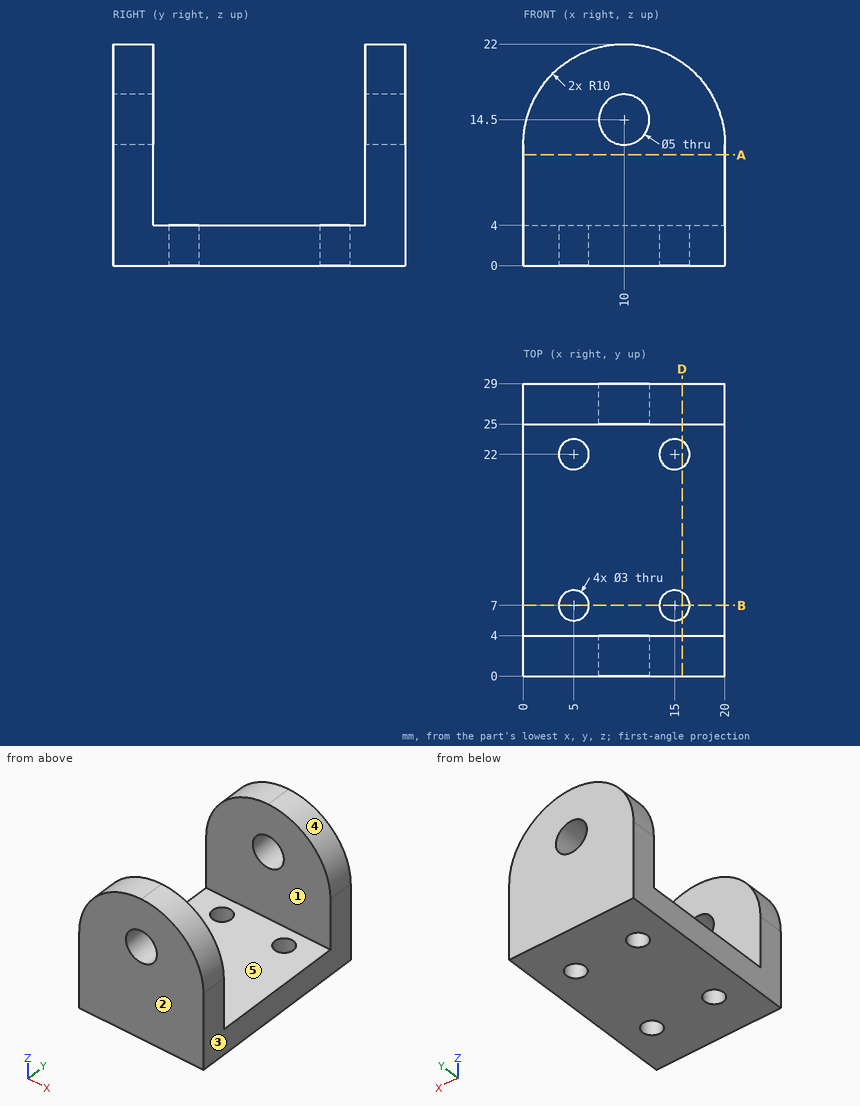
The figure shows three views and two pictorial views of one solid part (mm, origin at its lowest corner). Answer the questions. A direction names the side the tool comes from. Give positions to 0.01 mm unless a question says otherwise; leave off trailing zeros. Loops run counter-clockwise (first coordinate to the right, second up) from the corner with the lowest first, then second, coordinate; pieces in that order, holes last. Notation, with made-up numbers: (-14.5, 13) -> (19.5, 13) arc R24 cw to (19.5, 47) -> close; hole circle Ø9 at (52.5, 29.25). An arc over 180 degrees is marked (long way). Use a Markdown table: item, result. Add a question column.
1. Flat-ended cylindrical pins translate along their axes: pin 1 Ø8 at (y, z) = (8.5, 5) entering from +X; pin 2 Ø4 at (x, y) = (4, 8) entering from +Z. Find the tip coordinate at first contact, or state that the pin passes through.
2. Section A-A on z = 11 is taken. Determine the outline of the cut face in (x, y), and give its area (3 significant figures).
3. For the marked faces 4 and 5, determine the directions among +Z, -Z, +X, -X, +Y, -Y from which every point of the face is accessible in a straight line to the end or side of a thin tool.
4. Section D-D on x = 15.75 is taken. Determine the outline of the cut face in (y, z).
5. Section B-B on y = 7 is taken. Determine the outline of the cut face in (x, z), and give its area (3 significant figures).
6. Find the intervals of material crossed by probe 1 along Y at (x, z) = (5, 1.95); probe 2 along Z at (x, y) = (10, 26.75); probe 3 along Y at (x, z) = (4, 10.25), in increasing order.
7. Determine the mould class of the marked faces 1, 2 and 3 for opening direction Y: released by +Y, released by -Y, zero draft, split by the parting line, or undercut.
Results below:
| question | item | result |
|---|---|---|
| 1 | pin 1 | stops at x = 20 |
| 1 | pin 2 | stops at z = 4 |
| 2 | outline | (0, 0) -> (20, 0) -> (20, 4) -> (0, 4) -> close; (0, 25) -> (20, 25) -> (20, 29) -> (0, 29) -> close |
| 2 | area | 160 mm^2 |
| 3 | face 4 | +Z, +X, +Y, -Y |
| 3 | face 5 | +Z, +X, -X |
| 4 | outline | (0, 0) -> (5.7, 0) -> (5.7, 4) -> (4, 4) -> (4, 20.18) -> (0, 20.18) -> close; (8.3, 0) -> (20.7, 0) -> (20.7, 4) -> (8.3, 4) -> close; (23.3, 0) -> (29, 0) -> (29, 20.18) -> (25, 20.18) -> (25, 4) -> (23.3, 4) -> close |
| 5 | outline | (0, 0) -> (3.5, 0) -> (3.5, 4) -> (0, 4) -> close; (6.5, 0) -> (13.5, 0) -> (13.5, 4) -> (6.5, 4) -> close; (16.5, 0) -> (20, 0) -> (20, 4) -> (16.5, 4) -> close |
| 5 | area | 56.0 mm^2 |
| 6 | probe 1 | y = 0 to 5.5, 8.5 to 20.5, 23.5 to 29 |
| 6 | probe 2 | z = 0 to 12, 17 to 22 |
| 6 | probe 3 | y = 0 to 4, 25 to 29 |
| 7 | face 1 | undercut |
| 7 | face 2 | released by -Y |
| 7 | face 3 | zero draft |
